Check sheet for the drawn part. Datum: minimum x, y, z corner. Units: mm. A direction names the side the tool comes from. Coordinates: 2 decimals unless noted, no trailing zeros. Loops run counter-clockwise (first coordinate to the right, second up) from the corner with the lowest first, then second, coordinate; pieces in that order, holes last.
Q1. Sectioned sample at B-B (y = 84). Enter the section's corners in (x, z).
Q2. Sectioned sample at D-D (y = 26). Enter the section's corners in (x, z), then the cut area to 3 significant figures.
Q3. Go/stop test with flat-tipped pins: P1, Ø2, axis at y = 47.5, z = 99, coming from the +X side; P2, Ø6, axis at x = 30, y = 35, coming from the +Z side; P3, Ø4, axis at x = 8, z = 149, coming from the +Y side; P4, Ø1.5, axis at x = 15.5, y = 101.5, coming from the -Z side. Record where each tip stops, or that it passes through.
Q4. Sectioned sample at C-C (z = 191). Enter the section's corners in (x, y).
Q5. Sectioned sample at A-A (z = 129). Enter the section's corners in (x, y), then the cut area to 3 significant figures.
Q6. Material ranges on probe 1 along X at (y, z) = (103, 149); probe 2 along Y at (x, z) = (30, 1); probe 3 along Z at (x, y) = (52, 101), recorded low to high.
Q7. Access from +Z, -Z, +X, -X, +Y, -Y to the whole of each face (thin tool, end or side, straight path). Record for the marked faces 1, 2 and 3.
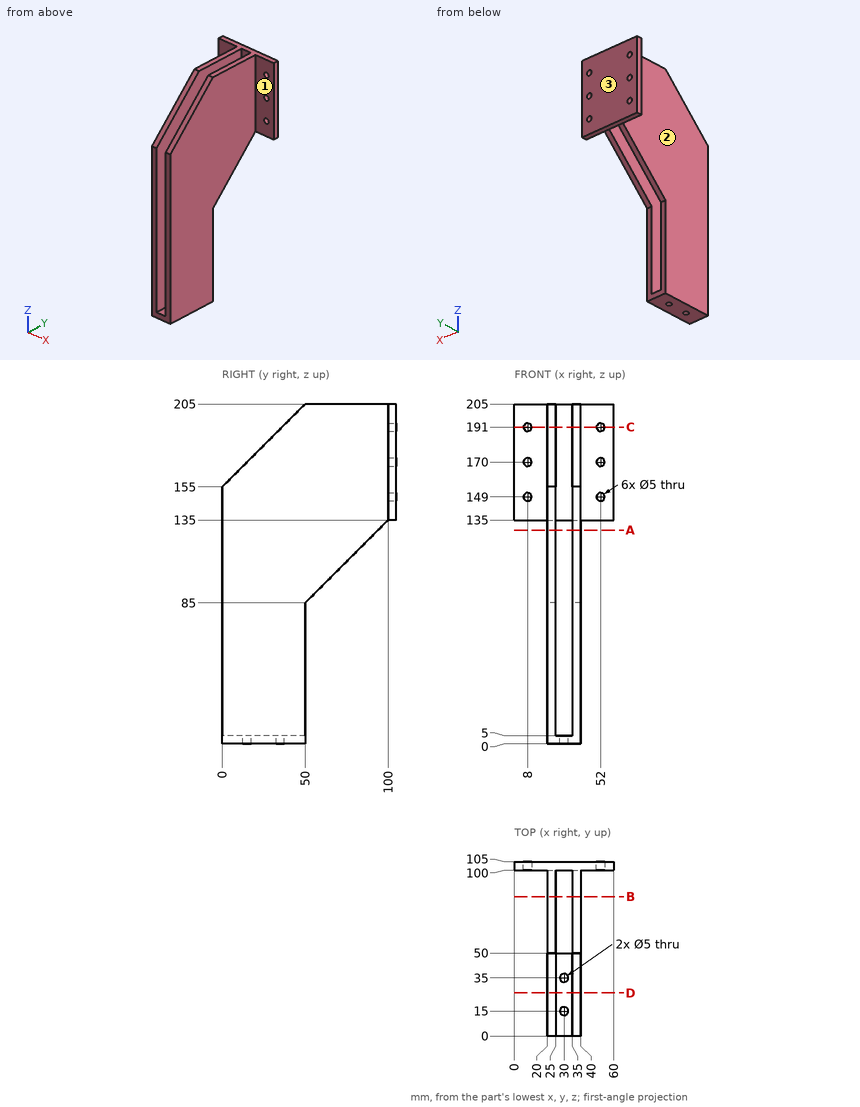
Geometry check:
1. outline: (20, 119) - (25, 119) - (25, 205) - (20, 205) - close; (35, 119) - (40, 119) - (40, 205) - (35, 205) - close
2. outline: (20, 0) - (40, 0) - (40, 181) - (35, 181) - (35, 5) - (25, 5) - (25, 181) - (20, 181) - close
2. area: 1,860 mm2
3. P1: stops at x = 40
3. P2: stops at z = 5
3. P3: passes through
3. P4: stops at z = 135
4. outline: (0, 100) - (5.5, 100) - (5.5, 105) - (0, 105) - close; (10.5, 100) - (20, 100) - (20, 36) - (25, 36) - (25, 100) - (35, 100) - (35, 36) - (40, 36) - (40, 100) - (49.5, 100) - (49.5, 105) - (10.5, 105) - close; (54.5, 100) - (60, 100) - (60, 105) - (54.5, 105) - close
5. outline: (20, 0) - (25, 0) - (25, 94) - (20, 94) - close; (35, 0) - (40, 0) - (40, 94) - (35, 94) - close
5. area: 940 mm2
6. probe 1: x = 0 to 5.5, 10.5 to 49.5, 54.5 to 60
6. probe 2: y = 0 to 12.5, 17.5 to 32.5, 37.5 to 50
6. probe 3: z = 135 to 146.5, 151.5 to 167.5, 172.5 to 188.5, 193.5 to 205
7. face 1: +Z, -Z, +X, -Y
7. face 2: +Z, -Z, -X, -Y
7. face 3: +Z, -Z, +X, -X, +Y
